```python
from build123d import *

# Parameters (mm, degrees)
CROQUIS1_R              = 1.8
CROQUIS1_R_2            = 1.5
CROQUIS1_R_3            = 1.75
SALIENTE_EXTRUIR1_DEPTH = 2


with BuildPart() as part:
    # Croquis1 → Saliente-Extruir1 (new body)
    with BuildSketch(Plane(origin=(0, 0, 0), x_dir=(1, 0, 0), z_dir=(0, 1, 0))):
        with BuildLine():
            Line((0.778192871, 2.897311833), (74.498192871, -16.903241843))
            ThreePointArc((74.498192871, -16.903241843), (76.10060692, -17.974982342), (76.72, -19.800553676))
            Line((76.72, -19.800553676), (76.72, -65.199446324))
            ThreePointArc((76.72, -65.199446324), (76.10060692, -67.025017658), (74.498192871, -68.096758157))
            Line((74.498192871, -68.096758157), (0.778192871, -87.897311833))
            ThreePointArc((0.778192871, -87.897311833), (-1.825571333, -87.38060692), (-3, -85))
            Line((-3, -85), (-3, 0))
            ThreePointArc((-3, 0), (-1.825571333, 2.38060692), (0.778192871, 2.897311833))
        make_face()
        with Locations(Location((25, -63.37, 0), (0, 0, 270))):
            Circle(CROQUIS1_R, mode=Mode.SUBTRACT)
        with Locations(Location((66.72, -21.65, 0), (0, 0, 270))):
            Circle(CROQUIS1_R, mode=Mode.SUBTRACT)
        with Locations(Location((66.72, -63.37, 0), (0, 0, 270))):
            Circle(CROQUIS1_R, mode=Mode.SUBTRACT)
        with Locations(Location((0, 0, 0), (0, 0, 270))):
            Circle(CROQUIS1_R_2, mode=Mode.SUBTRACT)
        with Locations(Location((0, -85, 0), (0, 0, 270))):
            Circle(CROQUIS1_R_2, mode=Mode.SUBTRACT)
        with Locations(Location((29, -19.1, 0), (0, 0, 270))):
            Circle(CROQUIS1_R_3, mode=Mode.SUBTRACT)
        with Locations(Location((61, -42.5, 0), (0, 0, 270))):
            Circle(CROQUIS1_R_3, mode=Mode.SUBTRACT)
    extrude(amount=SALIENTE_EXTRUIR1_DEPTH)


solid = part.part
```
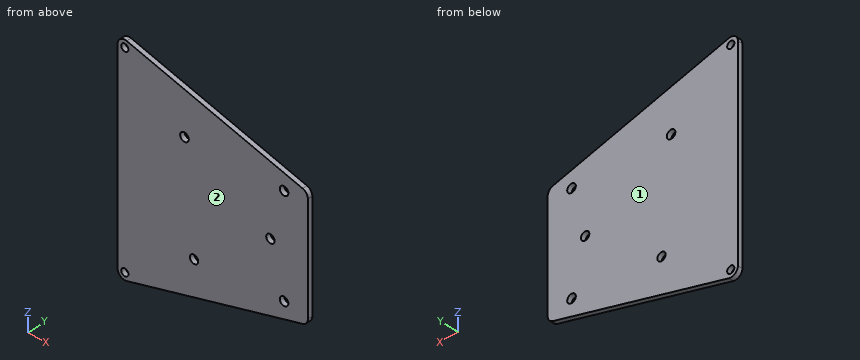
Input: part model. Units: mm. Frame: model coordinates. Face numbers are marked on the shaded views. Round coordinates to 2 decimals unless told otherwise and drop trailing zeros. Order: outer loops, then holes, each group sorted by start corner. A loop starts at its lowest first (then second) coordinate and runs counter-clockwise, first axis right, second up. Notation, with made-up numbers: (16, 13) - (43, 13) arc R11 cw to (43, 22) - close; hole circle Ø11 at (80, 34). An arc over 180 degrees is marked (long way). One line per question, with ' | ' between items. Start each with the question number.
1) Pull-direction query (Y, two-part tool) for the marked faces 1 and 2; classes: +Y half, -Y half, draft (parallel to the pull), parting line (faces both ways), or undercut.
2) Cut plane B-B, the plane z = 42.5. Return the cut outline in (x, y), then the cut area to 3 significant figures.
3) Ray query, probe 1 along X at (y, z) = (1.55, 42.5); probe 2 along X at (y, z) = (1.2, 63.37); probe 3 along Z at (x, y) = (66.72, 0.9). Return the intervals inside material, ascending.
4) Cut plane A-A, the plane z = 63.37. Return the cut outline in (x, y), then the cut area to 3 significant figures.
5) Contact query for a flat-ended pin moving along its axis: P1, Ø3, axis at x = 29, z = 19.1, coming from the -Y side. Output: stop coordinate, or through.
6) Cut plane C-C, the plane x = 61. Return the cut outline in (y, z), then the cut area to 3 significant figures.
7) Cut plane D-D, the plane y = 1.35. Return the cut outline in (x, z).
Worked out:
1) face 1: +Y half | face 2: -Y half
2) outline: (-3, 0) - (59.25, 0) - (59.25, 2) - (-3, 2) - close; (62.75, 0) - (76.72, 0) - (76.72, 2) - (62.75, 2) - close | area: 152 mm^2
3) probe 1: x = -3 to 59.25, 62.75 to 76.72 | probe 2: x = -3 to 23.2, 26.8 to 64.92, 68.52 to 76.72 | probe 3: z = 14.81 to 19.85, 23.45 to 61.57, 65.17 to 70.19
4) outline: (-3, 0) - (23.2, 0) - (23.2, 2) - (-3, 2) - close; (26.8, 0) - (64.92, 0) - (64.92, 2) - (26.8, 2) - close; (68.52, 0) - (76.72, 0) - (76.72, 2) - (68.52, 2) - close | area: 145 mm^2
5) P1: passes through
6) outline: (0, 13.28) - (2, 13.28) - (2, 40.75) - (0, 40.75) - close; (0, 44.25) - (2, 44.25) - (2, 71.72) - (0, 71.72) - close | area: 110 mm^2
7) outline: (-3, 0) arc R3 ccw to (0.78, -2.9) - (74.5, 16.9) arc R3 ccw to (76.72, 19.8) - (76.72, 65.2) arc R3 ccw to (74.5, 68.1) - (0.78, 87.9) arc R3 ccw to (-3, 85) - close; hole circle Ø3 at (0, 0); hole circle Ø3 at (0, 85); hole circle Ø3.6 at (25, 63.37); hole circle Ø3.5 at (29, 19.1); hole circle Ø3.5 at (61, 42.5); hole circle Ø3.6 at (66.72, 21.65); hole circle Ø3.6 at (66.72, 63.37)
